Model file for the job. Use its own axes, mm. A direction names the side the tool comes from. Give positions to 0.01 mm unless a question says otherwise; leave off trailing zeros. Order: outer loops, then holes, each group sorted by start corner. A loop starts at its lowest first (then second) coordinate and runs counter-clockwise, first axis right, second up. Notation, with made-up numbers: M 31,65.5 L 89,65.5 A23 cw 89,103.5 Z; hole C 35.5,87 d11. An arc over 180 degrees is marked long. Return JSON: item names as keys, results as strings. Group by question number.
1. 3-axis set-ups, long thin cutter, end or side, ignore diameter. For faces 1 (the face through (153, 45, 0)), 2 (the face through (38, 22.86, 6)), 3 (the face through (82, 13.97, 6)), 4 (the face through (68.544, 70.047, 5.635)), 5 (the face through (137, 0, 6)): which of +Z, -Z, +X, -X, +Y, -Y reach the whole face in a straight line?
2. Pin check, flat tips, straight feed: pin 1 (4 mm diameter, centred on y = 69.5, z = 6.5, fed in from -X); pin 2 (4 mm diameter, centred on y = 41.5, z = 6, fed in from -X). Stop position of each tip, or through.
3. Slice it at C-C on y = 29.5. List the corners of the cut face in (x, z), then the cut area to 3 significant figures.
4. Slice it at B-B on z = 7.25. List the corners of the cut face in (x, y).
5. Wall check: probe 1 along Y at (x, z) = (76, 6); probe 2 along Y at (x, z) = (65, 6.5); probe 3 along X at (y, z) = (63.5, 0.5). Give the ranges that are in metal, low to high. Write a range as [from, to].
6. Two-plate mould, pull along X, no slides. Class faces 6 (the face through (6.519, 82.026, 5.795)), 7 (the face through (86.106, 18, 6)), 8 (the face through (90.17, 70, 6)), 9 (the face through (153, 45, 11.43)): released by +X, released by -X, zero draft, split by the parting line, or undercut.
7. Slice it at A-A on x = 40. List the corners of the cut face in (y, z), then the cut area to 3 significant figures.
from build123d import *

# Parameters (mm, degrees)
SKETCH1_W           = 254
SKETCH1_H           = 88.9
BOSS_EXTRUDE1_DEPTH = 11.43
FILLET1_R           = 22.86
FILLET2_R           = 22.86
SKETCH2_W           = 11.43
SKETCH2_H           = 43.18
CUT_EXTRUDE1_DEPTH  = 120.65
SKETCH3_W           = 8.89
SKETCH3_H           = 8.89
CUT_EXTRUDE2_DEPTH  = 11.43
SKETCH4_W           = 19.05
SKETCH4_H           = 8.128
CUT_EXTRUDE3_DEPTH  = 11.43
CUT_EXTRUDE4_DEPTH  = 8.128


with BuildPart() as part:
    # Sketch1 → Boss-Extrude1 (new body)
    with BuildSketch(Plane.XY):
        with Locations((127, 44.45)):
            Rectangle(SKETCH1_W, SKETCH1_H)
    extrude(amount=BOSS_EXTRUDE1_DEPTH)

    # Fillet1
    fillet1_edges = [part.edges().sort_by_distance(p)[0] for p in [
        (0, 88.9, 5.715),
    ]]
    fillet(fillet1_edges, radius=FILLET1_R)

    # Fillet2
    fillet2_edges = [part.edges().sort_by_distance(p)[0] for p in [
        (0, 0, 5.715),
    ]]
    fillet(fillet2_edges, radius=FILLET2_R)

    # Sketch2 → Cut-Extrude1 (cut)
    with BuildSketch(Plane.ZY):
        with Locations((5.715, 44.45)):
            Rectangle(SKETCH2_W, SKETCH2_H)
    extrude(amount=-CUT_EXTRUDE1_DEPTH, mode=Mode.SUBTRACT)

    # Sketch3 → Cut-Extrude2 (cut)
    with BuildSketch(Plane.XY.offset(11.43)):
        with Locations((81.661, 18.415)):
            Rectangle(SKETCH3_W, SKETCH3_H)
    extrude(amount=-CUT_EXTRUDE2_DEPTH, mode=Mode.SUBTRACT)

    # Sketch4 → Cut-Extrude3 (cut)
    with BuildSketch(Plane.XY.offset(11.43)):
        with Locations((80.645, 70.104)):
            Rectangle(SKETCH4_W, SKETCH4_H)
    extrude(amount=-CUT_EXTRUDE3_DEPTH, mode=Mode.SUBTRACT)

    # Sketch6 → Cut-Extrude4 (cut)
    with BuildSketch(Plane.XZ.offset(-66.04)):
        Polygon((66.04, 0), (71.12, 11.43), (71.12, 0), align=None)
    extrude(amount=-CUT_EXTRUDE4_DEPTH, mode=Mode.SUBTRACT)


solid = part.part
Result:
{
 "1": {"face 1": "-Z, +X, -X, +Y, -Y", "face 2": "+Z, -Z, -X", "face 3": "+Z, -Z", "face 4": "-Z", "face 5": "+Z, -Z, +X, -X, -Y"},
 "2": {"pin 1": "stops at x = 0.05", "pin 2": "stops at x = 120.65"},
 "3": {"outline": "M 120.65,0 L 254,0 L 254,11.43 L 120.65,11.43 Z", "area": "1,520 mm2"},
 "4": {"outline": "M 0,22.86 A22.86 ccw 22.86,0 L 254,0 L 254,88.9 L 22.86,88.9 A22.86 ccw 0,66.04 L 69.26,66.04 L 69.26,74.17 L 90.17,74.17 L 90.17,66.04 L 120.65,66.04 L 120.65,22.86 L 86.11,22.86 L 86.11,13.97 L 77.22,13.97 L 77.22,22.86 Z"},
 "5": {"probe 1": "y = [0, 22.86], [74.17, 88.9]", "probe 2": "y = [0, 22.86], [66.04, 88.9]", "probe 3": "x = [120.65, 254]"},
 "6": {"face 6": "released by -X", "face 7": "undercut", "face 8": "undercut", "face 9": "zero draft"},
 "7": {"outline": "M 0,0 L 22.86,0 L 22.86,11.43 L 0,11.43 Z; M 66.04,0 L 88.9,0 L 88.9,11.43 L 66.04,11.43 Z", "area": "523 mm2"}
}
